Autodesk Inventor part; units mm, degrees
ref_plane "YZ Plane" through (0, 0, 0) normal (1, 0, 0) x (0, 1, 0)
ref_plane "XZ Plane" through (0, 0, 0) normal (0, 1, 0) x (-1, 0, 0)
ref_plane "XY Plane" through (0, 0, 0) normal (0, 0, 1) x (1, 0, 0)
sketch "Эскиз1" plane through (0, 0, 0) normal (0, 1, 0) x (-1, 0, 0)
  line L0 (-7.5, 20) -> (7.5, 20)
  line L1 (7.5, 20) -> (7.5, -20)
  line L2 (7.5, -20) -> (-7.5, -20)
  line L3 (-7.5, -20) -> (-7.5, 20)
  line L4 (-7.5, 20) -> (7.5, -20) construction
  line L5 (7.5, 20) -> (-7.5, -20) construction
  line L6 (-1.05, 20) -> (1.05, 20)
  line L7 (1.05, 20) -> (1.05, 10)
  line L8 (1.05, 10) -> (-1.05, 10)
  line L9 (-1.05, 10) -> (-1.05, 20)
  circle A0 centre (0, 7.1898) radius 3
  circle A1 centre (0, 7.1898) radius 2
  point P0 (0, 0)
  point P1 (0, 20)
  dimension "d0" = 40
  dimension "d1" = 15
  dimension "d2" = 2.1
  dimension "d3" = 10
  dimension "d7" = 6
  dimension "d8" = 4
extrude "Выдавливание1" add sketch "Эскиз1" along normal blind 12 contours L0 L9 A0 L7 L1 L2 L3 | L0 L7 A0 L9 | A0 L8 | L8 A0 | A1
sketch "Эскиз2" plane through (0, 12, 0) normal (0, 1, 0) x (1, 0, 0)
  line L0 (1.25, 20) -> (1.25, 12)
  line L1 (1.25, 12) -> (-1.25, 12)
  line L2 (-1.25, 12) -> (-1.25, 20)
  circle A0 centre (0, 9.2728) radius 3
  circle A1 centre (0, 9.2728) radius 1.25
  line L3 (7.5, -20) -> (7.5, 20)
  line L4 (7.5, 20) -> (-7.5, 20)
  line L5 (-7.5, 20) -> (-7.5, -20)
  line L6 (-7.5, -20) -> (7.5, -20)
  line L7 (-1.25, 20) -> (1.25, 20)
  point P0 (0, 20)
  dimension "d13" = 2.5
  dimension "d14" = 8
  dimension "d15" = 6
  dimension "d16" = 2.5
  dimension "d23" = 8
extrude "Выдавливание2" cut sketch "Эскиз2" against normal blind 6 contours L0 A0 L2 L4 | A0 L1 | L1 A0
mirror "Зеркальное отражение1" about plane through (0, 0, 0) normal (0, 0, 1) of "Выдавливание2"
sketch "Эскиз3" plane through (7.5, 0, 20) normal (1, 0, 0) x (0, 0, -1)
  line L0 (7, 3) -> (33, 3)
  line L1 (33, 3) -> (33, 0)
  line L2 (33, 0) -> (7, 0)
  line L3 (7, 0) -> (7, 3)
  line L4 (7, 3) -> (33, 0) construction
  line L5 (33, 3) -> (7, 0) construction
  line L6 (0, 0) -> (40, 0)
  point P0 (20, 0)
  point P1 (20, 1.5)
  point P2 (20, 0)
  dimension "d19" = 26
  dimension "d20" = 3
extrude "Выдавливание3" cut sketch "Эскиз3" against normal up to surface (15 mm away)
sketch "Эскиз4" plane through (0, 0, 0) normal (0, -1, 0) x (1, 0, 0)
  circle A0 centre (0, -25) radius 5
  circle A1 centre (0, -25) radius 1.6
  line L0 (7.5, 20) -> (7.5, -20)
  line L1 (7.5, -20) -> (4.6154, -26.9231)
  line L2 (-1.25, -20) -> (-7.5, -20)
  line L3 (-4.6154, -26.9231) -> (-7.5, -20)
  line L4 (7.5, -20) -> (-7.5, -20)
  point P0 (0, 0)
  dimension "d24" = 10
  dimension "d25" = 3.2
extrude "Выдавливание4" add sketch "Эскиз4" against normal blind 3
sketch "Эскиз5" plane through (0, 3, 0) normal (0, 1, 0) x (1, 0, 0)
  circle A0 centre (0, 25) radius 1.6
  arc A1 (4.6154, 26.9231) -> (-4.6154, 26.9231) centre (0, 25) ccw
  line L0 (-3.1186, 25.5982) -> (-1.0412, 27.9999)
  line L1 (-1.0412, 27.9999) -> (2.0774, 27.4016)
  line L2 (2.0774, 27.4016) -> (3.1186, 24.4018)
  line L3 (3.1186, 24.4018) -> (1.0412, 22.0001)
  line L4 (1.0412, 22.0001) -> (-2.0774, 22.5984)
  line L5 (-2.0774, 22.5984) -> (-3.1186, 25.5982)
  point P0 (0, 0)
  point P1 (-2.598, 24.0983)
  point P2 (2.598, 25.9017)
  dimension "d32" = 5.5
extrude "Выдавливание5" cut sketch "Эскиз5" against normal blind 2.3
mirror "Зеркальное отражение2" about plane through (0, 0, 0) normal (0, 0, 1) of "Выдавливание4", "Выдавливание5"
fillet "Сопряжение1" radius 3 4 edges at (-1.25, 9, -12) (1.25, 9, -12) (-1.25, 9, 12) (1.25, 9, 12)
properties part number "крепление_ремня_новое"
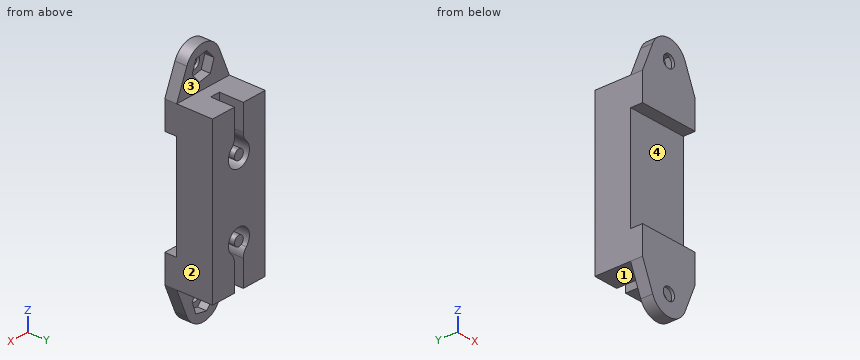
For this review, take the finished solid that the model builds, in its own axes (mm). Face numbers are marked on the shaded views. A direction names the side the tool comes from. Give positions to 0.01 mm unless a question says otherwise; leave off trailing zeros. Loops run counter-clockwise (first coordinate to the right, second up) from the corner with the lowest first, then second, coordinate; pieces in that order, holes last. Notation, with made-up numbers: M -4,59.5 L 21,59.5 A24 ccw 21,88.5 Z; hole C -4,11 d7. An arc over 180 degrees is marked long. Put each result on its own line as item: value. Start each with the question number.
(1) Add section D-D, the plane x = 0. Give the number of separate pieces and of enclosed holes in the cut face, then the cut area to 3 significant figures.
(2) Add section B-B, the plane y = 10. Write out the cut boundary in (x, z) (3 decimals).
(3) Add section C-C, the plane z = -25. Write out the cut boundary in (x, y), then the cut area to 3 significant figures.
(4) Add section A-A, the plane z = -18. Write out the cut boundary in (x, y).
(5) Wall thickness on L1, parallel to Z at x = 0, y = 9.8; L2, parallel to Z at x = 0, y = 0.4; L3, parallel to X at y = 6.5, z = -9: over which ranges is each line inside the solid? List them lowest first.
(6) For pin 1 (6.5 mm diameter, centred on x = -0.5, z = -26, fed in from +Y); pin 2 (1 mm diameter, centred on x = 1, y = 6, fed in from +Z); pin 3 (6 mm diameter, centred on x = 3.5, z = -0.5, fed in from -Y), all flat-tipped, find the tip position at first contact; note any pin that passes through.
(7) Machinability: for the marked faces 1, 2, 3 and 4, which of the approach directions +Z, -Z, +X, -X, +Y, -Y give a long, thin tool a straight path to every point of the face, cutting with its end or side? Answer none if there is none.
Result:
1. separate pieces: 3
1. enclosed holes: 0
1. area: 297 mm^2
2. outline: M -7.5,-20 L -1.25,-20 L -1.25,-13.508 A3 ccw -2.125,-11.39 A3 cw long 2.125,-11.39 A3 ccw 1.25,-13.508 L 1.25,-20 L 7.5,-20 L 7.5,20 L 1.25,20 L 1.25,13.508 A3 ccw 2.125,11.39 A3 cw long -2.125,11.39 A3 ccw -1.25,13.508 L -1.25,20 L -7.5,20 Z; C 0,-9.273 d2.5; C 0,9.273 d2.5
3. outline: M -5.42,0 L -1.6,0 L -1.6,0.7 L -2.91,0.7 L -2.91,3 L -5.42,3 Z; M 1.6,0 L 5.42,0 L 5.42,3 L 2.91,3 L 2.91,0.7 L 1.6,0.7 Z
3. area: 16.9 mm^2
4. outline: M -7.5,0 L 7.5,0 L 7.5,12 L 1.25,12 L 1.25,6 L -1.25,6 L -1.25,12 L -7.5,12 Z
5. L1: z = -10.52 to -8.02, -6.27 to 6.27, 8.02 to 10.52
5. L2: z = -30 to -26.6, -23.4 to -13, 13 to 23.4, 26.6 to 30
5. L3: x = -7.5 to -2.99, -1.22 to 1.22, 2.99 to 7.5
6. pin 1: stops at y = 3
6. pin 2: stops at z = 20
6. pin 3: stops at y = 3
7. face 1: -Z, +X, -X, +Y
7. face 2: +Z, -Z, +X, +Y, -Y
7. face 3: +Z, +X, -X, +Y
7. face 4: +X, -X, -Y
